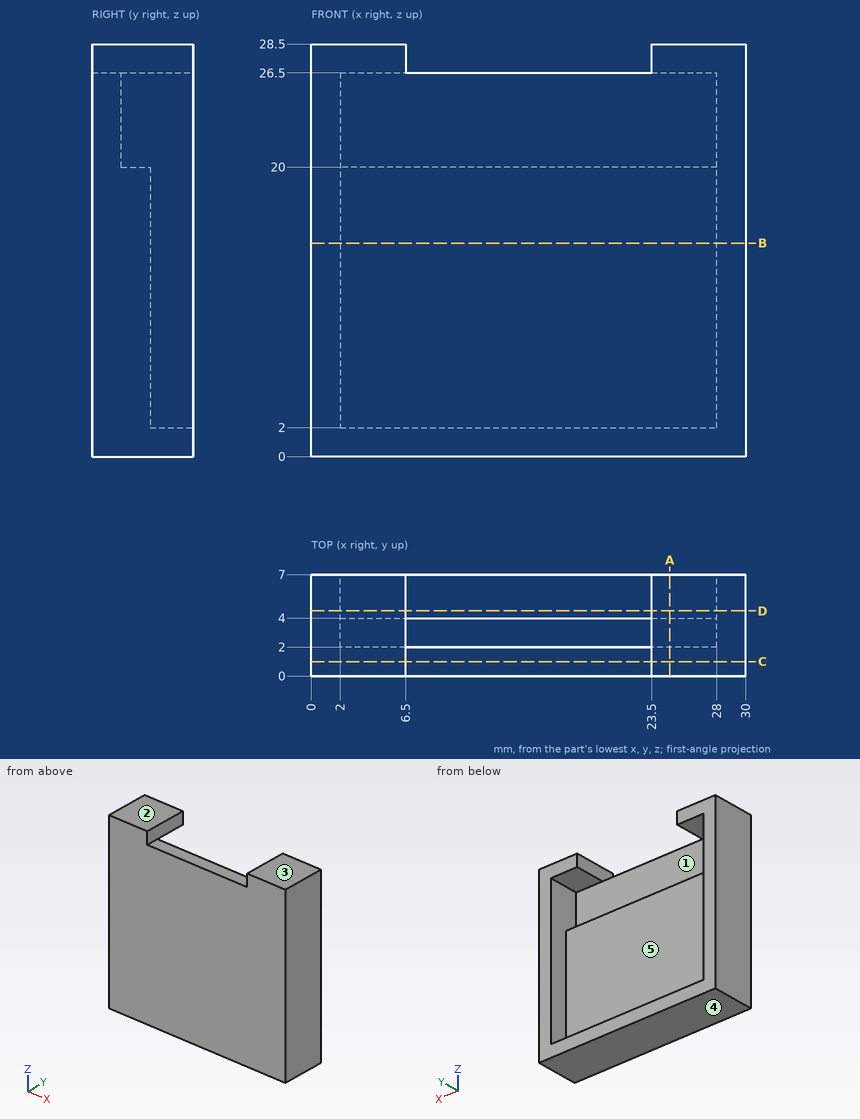
Check sheet for the drawn part. Datum: minimum x, y, z corner. Units: mm. A direction names the side the tool comes from. Coordinates: 2 decimals unless noted, no trailing zeros. Order: outer loops, then holes, each group sorted by start corner. A loop starts at its lowest first (then second) coordinate and runs counter-clockwise, first axis right, second up. Notation, with made-up numbers: M 33.25,-7.75 L 87.25,-7.75 A20 cw 87.25,7.25 Z; hole C -16.5,34.5 d3. An arc over 180 degrees is marked long. One line per question, with ' | ' between items. Start each with the question number.
Item 1: Material ranges on line 1 (X direction, y = 4.25, z = 21); line 2 (Z direction, x = 5.75, y = 5); line 3 (Y direction, x = 2.5, z = 25.5), recorded low to high.
Item 2: Sectioned sample at C-C on y = 1. Record the cut outline in (x, z), and give its area (3 significant figures).
Item 3: Access from +Z, -Z, +X, -X, +Y, -Y to the whole of each face (thin tool, end or side, straight path). Record for the marked faces 1 and 2.
Item 4: Sectioned sample at A-A on x = 24.75. Record the cut outline in (y, z), and give its area (3 significant figures).
Item 5: Sectioned sample at D-D on y = 4.5. Record the cut outline in (x, z).
Item 6: Gauge pin test, flat ends, axial feed: P1, Ø3, axis at x = 13.5, z = 16.5, coming from the +Y side; P2, Ø2, axis at x = 11.5, y = 1, coming from the +Z side; P3, Ø1.5, axis at x = 12.5, y = 6, coming from the +Z side. Record the tip position at first contact, or that the pin passes through.
Item 7: Mould release check, pull along Z, two halves, no side actions. Record for the marked faces 3, 4 and 5: pulls with the +Z half, pulls with the -Z half, needs draft (parallel to the pull), parting line crosses it, or undercut.
Item 8: Sectioned sample at B-B on z = 14.75. Record the cut outline in (x, y), and give its area (3 significant figures).
Answer below:
1) line 1: x = 0 to 2, 28 to 30 | line 2: z = 0 to 2, 26.5 to 28.5 | line 3: y = 0 to 2
2) outline: M 0,0 L 30,0 L 30,28.5 L 23.5,28.5 L 23.5,26.5 L 6.5,26.5 L 6.5,28.5 L 0,28.5 Z | area: 821 mm^2
3) face 1: +Y | face 2: +Z, +X, -X, +Y, -Y
4) outline: M 0,0 L 7,0 L 7,2 L 4,2 L 4,20 L 2,20 L 2,26.5 L 7,26.5 L 7,28.5 L 0,28.5 Z | area: 113 mm^2
5) outline: M 0,0 L 30,0 L 30,28.5 L 23.5,28.5 L 23.5,26.5 L 28,26.5 L 28,2 L 2,2 L 2,26.5 L 6.5,26.5 L 6.5,28.5 L 0,28.5 Z
6) P1: stops at y = 4 | P2: stops at z = 26.5 | P3: stops at z = 2
7) face 3: pulls with the +Z half | face 4: pulls with the -Z half | face 5: undercut
8) outline: M 0,0 L 30,0 L 30,7 L 28,7 L 28,4 L 2,4 L 2,7 L 0,7 Z | area: 132 mm^2
